Could you check a few things on this model? Use its own coordinates, in mm. A direction names the side the tool comes from. Round coordinates to 2 decimals unless told otherwise and drop trailing zeros. Order: outer loops, then holes, each group sorted by start corner. A loop starts at its lowest first (then second) coordinate and runs counter-clockwise, first axis right, second up.
```python
from build123d import *

# Parameters (mm, degrees)
F1_DEPTH = 15
F2_R     = 13
F3_DEPTH = 30.001
F4_W     = 14
F4_H     = 4
F5_DEPTH = 11.001
F6_R     = 7
F7_DEPTH = 68.001


# Not quite as in the source:
# - a pattern or mirror of a feature is missing from the dataset's text; its kind, count and spacing are read off the source's solid


with BuildPart() as f1:
    # F0 (on Right) → F1 (new body, symmetric)
    with BuildSketch(Plane.YZ):
        Polygon((-17, 0), (0, 0), (17, 0), (17, 5), (40, 5), (40, 11), (28, 11), (28, 35), (18, 35), (10, 40), (0, 40), (-10, 40), (-18, 35), (-28, 35), (-28, 11), (-40, 11), (-40, 5), (-17, 5), align=None)
    extrude(amount=F1_DEPTH, both=True)

    # F2 (on face) → F3 (cut, through all)
    with BuildSketch(Plane.YZ.offset(15)):
        with Locations((0, 21)):
            Circle(F2_R)
    extrude(amount=-F3_DEPTH, mode=Mode.SUBTRACT)

    # F4 (on face) → F5 (cut, through all)
    with BuildSketch(Plane.XY.offset(11)):
        with Locations((0, -38)):
            Rectangle(F4_W, F4_H)
    f5 = extrude(amount=-F5_DEPTH, mode=Mode.SUBTRACT)

    # F5_copies: F5 across plane
    add(f5.mirror(Plane.ZX), mode=Mode.SUBTRACT)

    # F6 (on face) → F7 (cut, through all)
    with BuildSketch(Plane.XZ.offset(28)):
        with Locations((0, 25)):
            Circle(F6_R)
    extrude(amount=-F7_DEPTH, mode=Mode.SUBTRACT)


solid = f1.part
```
Q1. Imagine slicing it at B-B, the plane x = 11. Please give me the cut outline in (y, z).
Q2. Imagine slicing it at C-C, the plane z = 21. Please give me the cut outline in (x, y), then the cut area to 3 significant figures.
Q3. Imagine slicing it at D-D, the plane x = 1. Please give me the cut outline in (y, z).
Q4. For faces 5 (the flat face through (0, -23, 35)), 6 (the flat face through (0, 28, 17)), 7 (the flat face through (7, 38, 8)), 8 (the flat face through (-7, -38, 8)), which set-ups out of +Z, -Z, +X, -X, +Y, -Y let a thin tool reach every point of the face, with its end or its side?
Q5. We'd pull the mould along X, two halves only. Please class faces 1 (the cylindrical face through (-0.91, 19.66, 31.94)), 2 (the flat face through (15, -9, 11)), 3 (the flat face through (0, -17, 3)), 4 (the flat face through (0, -36, 8)): released by +X, released by -X, zero draft, split by the parting line, or undercut.
Q6. I need wall thicknesses on L1, parallel to X at y = 21.5, z = 25; L2, parallel to Z at x = 10, y = 0.5; L3, parallel to Y at x = -2, z = 6.5. Which ranges of each line are inside material? Lowest first, please.
Q7. For P1, Ø7, axis at x = -4.5, y = -26, coming from the -Z side; P2, Ø10, axis at x = 2.5, z = 22, coming from the -Y side; P3, Ø5, axis at x = -5, y = -21, coming from the +Z side, each with a flat end and sliding along its axis, tell me the tip position at first contact or that it passes through.
Q8. Imagine slicing it at A-A, the plane y = 0. Please give me the cut outline in (x, z), then the cut area to 3 significant figures.
Filled in:
1. outline: (-40, 5) - (-17, 5) - (-17, 0) - (17, 0) - (17, 5) - (40, 5) - (40, 11) - (28, 11) - (28, 35) - (18, 35) - (10, 40) - (-10, 40) - (-18, 35) - (-28, 35) - (-28, 11) - (-40, 11) - close; hole circle Ø26 at (0, 21)
2. outline: (-15, -28) - (-5.74, -28) - (-5.74, -13) - (-15, -13) - close; (-15, 13) - (-5.74, 13) - (-5.74, 28) - (-15, 28) - close; (5.74, -28) - (15, -28) - (15, -13) - (5.74, -13) - close; (5.74, 13) - (15, 13) - (15, 28) - (5.74, 28) - close
2. area: 555 mm2
3. outline: (-36, 5) - (-17, 5) - (-17, 0) - (17, 0) - (17, 5) - (36, 5) - (36, 11) - (28, 11) - (28, 18.07) - (12.67, 18.07) arc R13 cw to (-12.67, 18.07) - (-28, 18.07) - (-28, 11) - (-36, 11) - close; (-28, 31.93) - (-7.04, 31.93) arc R13 cw to (7.04, 31.93) - (28, 31.93) - (28, 35) - (18, 35) - (10, 40) - (-10, 40) - (-18, 35) - (-28, 35) - close
4. face 5: +Z, +X, -X, -Y
4. face 6: +Z, +X, -X, +Y
4. face 7: +Z, -Z, +Y
4. face 8: +Z, -Z, -Y
5. face 1: undercut
5. face 2: released by +X
5. face 3: zero draft
5. face 4: undercut
6. L1: x = -15 to -7, 7 to 15
6. L2: z = 0 to 8.01, 33.99 to 40
6. L3: y = -36 to 36
7. P1: stops at z = 5
7. P2: stops at y = -28
7. P3: stops at z = 35
8. outline: (-15, 0) - (15, 0) - (15, 8) - (-15, 8) - close; (-15, 34) - (15, 34) - (15, 40) - (-15, 40) - close
8. area: 420 mm2
